Geometry check sheet. Reference: the model listing, model coordinates, mm. A direction names the side the tool comes from. Round coordinates to 2 decimals unless told otherwise and drop trailing zeros. Write each loop counter-clockwise with the first axis right and the second up, starting at its lowest first coordinate (ties: lowest second). Pieces come first, ordered by that corner, then holes. Notation, with made-up numbers: (13, -13.75) - (33, -13.75) arc R10 cw to (33, 2.25) - close; hole circle Ø1 at (39.25, 18). An arc over 180 degrees is marked (long way). Return JSON: item names as keys, results as strings.
Autodesk Inventor part; units mm, degrees
ref_plane "YZ Plane" through (0, 0, 0) normal (1, 0, 0) x (0, 1, 0)
ref_plane "XZ Plane" through (0, 0, 0) normal (0, 1, 0) x (-1, 0, 0)
ref_plane "XY Plane" through (0, 0, 0) normal (0, 0, 1) x (1, 0, 0)
sketch "Sketch1" plane through (0, 0, 0) normal (0, 0, 1) x (1, 0, 0)
  line L0 (0, 0) -> (0, 110)
  line L1 (0, 110) -> (110, 110)
  line L2 (110, 110) -> (110, 0)
  line L3 (110, 0) -> (0, 0)
  dimension "d0" = 110
  dimension "d1" = 110
extrude "Extrusion1" add sketch "Sketch1" along normal blind 3
sketch "Sketch2" plane through (0, 0, 0) normal (0, 0, -1) x (-1, 0, 0)
  line L0 (0, 0) -> (3, 0)
  line L1 (3, 0) -> (3, 113)
  line L2 (3, 113) -> (-113, 113)
  line L3 (-113, 113) -> (-113, -3)
  line L4 (-113, -3) -> (3, -3)
  line L5 (3, -3) -> (3, 0)
  line L6 (-110, 110) -> (0, 110)
  line L7 (0, 110) -> (0, 0)
  line L8 (0, 0) -> (-110, 0)
  line L9 (-110, 0) -> (-110, 110)
  dimension "d4" = 3
  dimension "d5" = 113
  dimension "d6" = 116
  dimension "d7" = 116
extrude "Extrusion2" add sketch "Sketch2" against normal blind 40
sketch "Sketch3" plane through (0, 0, 3) normal (0, 0, 1) x (1, 0, 0)
  line L0 (110, 0) -> (0, 0)
  line L1 (55, 0) -> (55, 5)
  line L2 (55, 5) -> (10, 5)
  line L3 (55, 5) -> (100, 5)
  line L4 (100, 5) -> (100, 99)
  line L5 (100, 99) -> (10, 99)
  line L6 (10, 99) -> (10, 5)
  circle A0 centre (10, 5) radius 3.5
  circle A1 centre (10, 99) radius 3.5
  circle A2 centre (100, 99) radius 3.5
  circle A3 centre (100, 5) radius 3.5
  dimension "d10" = 5
  dimension "d11" = 45
  dimension "d12" = 45
  dimension "d13" = 94
  dimension "d14" = 90
  dimension "d15" = 7
  dimension "d16" = 7
  dimension "d17" = 7
  dimension "d18" = 7
extrude "Extrusion3" add sketch "Sketch3" along normal blind 20 contours A0 L6 L2 | L2 L6 A0 | A3 L4 L3 | L3 L4 A3 | A1 L5 L6 | L6 L5 A1 | A2 L5 L4 | L4 L5 A2
sketch "Sketch4" plane through (10, 99, 23) normal (0, 0, 1) x (1, 0, 0)
  circle A0 centre (0, 0) radius 1.75
  circle A1 centre (90, 0) radius 3.5
  circle A2 centre (90, 0) radius 1.75
  circle A3 centre (90, -94) radius 3.5
  circle A4 centre (90, -94) radius 1.75
  circle A5 centre (0, -94) radius 3.5
  circle A6 centre (0, -94) radius 1.75
  point P0 (-10, -99)
  point P1 (90, -99)
  point P2 (0, -99)
  dimension "d21" = 3.5
  dimension "d22" = 3.5
  dimension "d23" = 3.5
extrude "Extrusion4" cut sketch "Sketch4" against normal through all contours A0 | A2 | A4 | A6
sketch "Sketch5" plane through (0, 0, 3) normal (0, 0, 1) x (1, 0, 0)
  line L0 (110, 0) -> (0, 0)
  line L1 (55, 0) -> (55, 20)
  line L2 (55, 20) -> (85, 20)
  line L3 (85, 20) -> (85, 80)
  line L4 (85, 80) -> (25, 80)
  line L5 (25, 80) -> (25, 20)
  circle A0 centre (25, 20) radius 1.75
  circle A1 centre (25, 80) radius 1.75
  circle A2 centre (85, 80) radius 1.75
  circle A3 centre (85, 20) radius 1.75
  dimension "d26" = 20
  dimension "d27" = 30
  dimension "d28" = 60
  dimension "d29" = 60
  dimension "d30" = 3.5
  dimension "d31" = 3.5
  dimension "d32" = 3.5
  dimension "d33" = 3.5
extrude "Extrusion5" cut sketch "Sketch5" against normal through all
chamfer "Chamfer1" distance 4 angle 45 4 edges at (6.5, 99, 3) (96.5, 99, 3) (6.5, 5, 3) (96.5, 5, 3)
sketch "Sketch6" plane through (113, -3, 0) normal (1, 0, 0) x (0, 0, -1)
  line L0 (-23, 105.5) -> (-23, 98.5)
  line L1 (-23, 105.738) -> (-37, 105.738)
  line L2 (-23, 105.738) -> (-9, 105.738) construction
  line L3 (-23, 11.5) -> (-23, 4.5)
  line L4 (-23, 4.3379) -> (-37, 4.3379)
  line L5 (-23, 4.3379) -> (-9, 4.3379) construction
  line L6 (-37, 4.3379) -> (-37, 105.738)
  line L7 (-23, 105.738) -> (-23, 85.738)
  line L8 (-23, 85.738) -> (-8, 85.738)
  line L9 (-8, 85.738) -> (-8, 35.738)
  line L10 (-8, 35.738) -> (-23, 35.738)
  line L11 (-23, 35.738) -> (-23, 4.3379)
  point P0 (0, 3)
  dimension "d39" = 14
  dimension "d40" = 180
  dimension "d41" = 14
  dimension "d42" = 180
  dimension "d43" = 20
  dimension "d44" = 15
  dimension "d45" = 50
extrude "Extrusion6" cut sketch "Sketch6" against normal up to surface (3 mm away)
sketch "Sketch7" plane through (-3, -3, 0) normal (-1, 0, 0) x (0, 0, 1)
  line L0 (23, 105.738) -> (33, 105.738)
  line L1 (33, 105.738) -> (33, 5.738)
  line L2 (33, 5.738) -> (23, 5.738)
  line L3 (23, 5.738) -> (23, 105.738)
  point P0 (0, 3)
  dimension "d48" = 10
  dimension "d49" = 100
extrude "Extrusion7" cut sketch "Sketch7" against normal up to surface (3 mm away)
sketch "Sketch8" plane through (0, 0, 0) normal (0, 0, -1) x (-1, 0, 0)
  circle A0 centre (-10, 5) radius 1.75
  line L0 (-10, 5) -> (-20, 5)
  line L1 (-20, 5) -> (-20, 7)
  line L2 (-20, 5) -> (-18, 5) construction
  circle A1 centre (-20, 7) radius 5
  point P0 (0, 0)
  dimension "d52" = 10
  dimension "d53" = 2
  dimension "d54" = 90
  dimension "d55" = 10
extrude "Extrusion8" cut sketch "Sketch8" against normal blind 20 contours A1
equation "\"d15\" = d16"
equation "\"d17\" = d16"
equation "\"d18\" = d16"
properties part number "nuccase"
(1) Section check C-C, the plane z = 29. Enter the section's corners in (x, y), plus the area to 3 significant figures.
Response values:
{"outline": "(-3, -3) - (113, -3) - (113, 1.34) - (110, 1.34) - (110, 0) - (0, 0) - (0, 2.74) - (-3, 2.74) - close; (-3, 102.74) - (0, 102.74) - (0, 110) - (110, 110) - (110, 102.74) - (113, 102.74) - (113, 113) - (-3, 113) - close", "area": "752 mm^2"}
(2) Material ranges on line 1 along X through (y, z) = (80, 1.4); line 2 along X through (y, z) = (99, 16); line 3 along Y through (x, z) = (100, 9.25), recorded low to high. Write a range as [from, to].
Response values:
{"line 1": "x = [-3, 23.25], [26.75, 83.25], [86.75, 113]", "line 2": "x = [-3, 0], [6.5, 8.25], [11.75, 13.5], [96.5, 98.25], [101.75, 103.5], [110, 113]", "line 3": "y = [-3, 0], [1.5, 3.25], [6.75, 8.5], [95.5, 97.25], [100.75, 102.5], [110, 113]"}
(3) Section check D-D, the plane x = 20. Enter the section's corners in (y, z), plus the area to 3 significant figures.
Response values:
{"outline": "(-3, 0) - (2, 0) - (2, 3) - (0, 3) - (0, 40) - (-3, 40) - close; (12, 0) - (113, 0) - (113, 40) - (110, 40) - (110, 3) - (12, 3) - close", "area": "540 mm^2"}
(4) Section check A-A, the plane x = 85. Enter the section's corners in (y, z), plus the area to 3 significant figures.
Response values:
{"outline": "(-3, 0) - (18.25, 0) - (18.25, 3) - (0, 3) - (0, 40) - (-3, 40) - close; (21.75, 0) - (78.25, 0) - (78.25, 3) - (21.75, 3) - close; (81.75, 0) - (113, 0) - (113, 40) - (110, 40) - (110, 3) - (81.75, 3) - close", "area": "549 mm^2"}
(5) Access from +Z, -Z, +X, -X, +Y, -Y to the whole of each face (thin tool, end or side, straight path). Record for faces 1 (the face through (54, 0, 21)), 2 (the face through (8, 4, 23)), 3 (the face through (-2, 2.738, 28)), 4 (the face through (24.62, 78.29, 1.52)).
Response values:
{"face 1": "+Z", "face 2": "+Z, +X", "face 3": "+X, -X", "face 4": "+Z, -Z"}
(6) Gauge pin test, flat ends, axial feed: pin 1 (8 mm diameter, centred on x = 38.5, y = 19.5, fed in from +Z); pin 2 (18.5 mm diameter, centred on y = 70, z = 21, fed in from +X); pin 3 (7.5 mm diameter, centred on x = 101, y = 100, fed in from +Z). Record the tip position at first contact, or that the pin passes through.
Response values:
{"pin 1": "stops at z = 3", "pin 2": "stops at x = 0", "pin 3": "stops at z = 23"}
(7) Section check B-B, the plane y = 20. Enter the section's corners in (x, z), plus the area to 3 significant figures.
Response values:
{"outline": "(-3, 0) - (23.25, 0) - (23.25, 3) - (0, 3) - (0, 23) - (-3, 23) - close; (-3, 33) - (0, 33) - (0, 40) - (-3, 40) - close; (26.75, 0) - (83.25, 0) - (83.25, 3) - (26.75, 3) - close; (86.75, 0) - (113, 0) - (113, 23) - (110, 23) - (110, 3) - (86.75, 3) - close; (110, 37) - (113, 37) - (113, 40) - (110, 40) - close", "area": "477 mm^2"}
(8) Release check for a two-part mould opening along X. For faces 5 (the face through (6.503, 4.846, 14.888)), 6 (the face through (103.233, 6.341, 14.888)), 7 (the face through (-3, 54, 20)), 8 (the face through (112, 17, 23)) record: pulls with the +X half, pulls with the -X half, needs draft (parallel to the pull), parting line crosses it, or undercut.
Response values:
{"face 5": "undercut", "face 6": "undercut", "face 7": "pulls with the -X half", "face 8": "needs draft"}
